The listing builds one solid part. Answer for the finished solid, in the listing's coordinates (mm). A direction names the side the tool comes from. Round coordinates to 2 decimals unless told otherwise and drop trailing zeros. Write each loop counter-clockwise with the first axis right and the second up, starting at its lowest first coordinate (ties: lowest second). Pieces come first, ordered by that corner, then holes.
(1) A cutting plane is placed at C-C, the plane y = 6. Give the vertices of the cut face in (x, z), and give its area (3 significant figures).
(2) For faces 4 (the face through (-2, 16.7, -3.5)), 5 (the face through (-3.4, 11.3, -5)), 6 (the face through (-8, 3.7, -4)), 7 (the face through (-7.5, 1.9, 6.5)), determine the directions among +Z, -Z, +X, -X, +Y, -Y from which every point of the face is accessible in a straight line to the end or side of a thin tool.
(3) A cutting plane is placed at D-D, the plane x = -1.75. Give the vertices of the cut face in (y, z), and give its area (3 significant figures).
(4) A cutting plane is placed at A-A, the plane z = 1.5. Give the vertices of the cut face in (x, y).
(5) Find the intervals of material crossed by probe 1 along X at (y, z) = (1.5, 1.25); probe 2 along X at (y, z) = (11.5, -4.25); probe 3 along X at (y, z) = (10, -5.5), in increasing order.
(6) Each of these flat-tipped pins is pushed along its axis until it touches: pin 1 Ø6.5 at (y, z) = (7.5, -5) entering from +X; pin 2 Ø3.5 at (x, y) = (-4.5, 12) entering from -Z; pin 3 Ø0.9 at (x, z) = (-7.5, -4) entering from -Y. Where does it stop, or does it pass through?
(7) A cutting plane is placed at B-B, the plane x = -7.5. Give the vertices of the cut face in (y, z).
(8) The mould has two halves that part along X. Classify faces 1 (the face through (6.55, 2, 0)), 2 (the face through (-4, 11, -2)), 3 (the face through (-10.5, 7, -3)): +X half, -X half, draft (parallel to the pull), parting line (faces both ways), or undercut.
from build123d import *

# Parameters (mm, degrees)
SKETCH1_W           = 10
SKETCH1_H           = 16
BOSS_EXTRUDE1_DEPTH = 3.7
SKETCH5_W           = 5.5
SKETCH5_H           = 16
BOSS_EXTRUDE2_DEPTH = 3.7
CUT_EXTRUDE4_DEPTH  = 4.7
BOSS_EXTRUDE3_START = -2
SKETCH7_W           = 17
SKETCH7_H           = 15
BOSS_EXTRUDE3_DEPTH = 3
SKETCH8_W           = 2.5
SKETCH8_H           = 15
BOSS_EXTRUDE5_DEPTH = 3


with BuildPart() as part:
    # Sketch1 → Boss-Extrude1 (new body)
    with BuildSketch(Plane(origin=(0, 0, 0), x_dir=(1, 0, 0), z_dir=(0, 1, 0))):
        Rectangle(SKETCH1_W, SKETCH1_H)
    extrude(amount=BOSS_EXTRUDE1_DEPTH)

    # Sketch5 → Boss-Extrude2 (add)
    with BuildSketch(Plane.XZ):
        with Locations((-7.75, 0)):
            Rectangle(SKETCH5_W, SKETCH5_H)
    boss_extrude2 = extrude(amount=-BOSS_EXTRUDE2_DEPTH)

    # Sketch6 → Cut-Extrude4 (cut, through all)
    with BuildSketch(Plane(origin=(0, 3.7, 0), x_dir=(1, 0, 0), z_dir=(0, 1, 0))):
        with BuildLine():
            Line((-6.55, 5.55), (-6.55, -5.55))
            ThreePointArc((-6.55, -5.55), (-7.5, -6.5), (-8.45, -5.55))
            Line((-8.45, -5.55), (-8.45, 5.55))
            ThreePointArc((-8.45, 5.55), (-7.5, 6.5), (-6.55, 5.55))
        make_face()
    cut_extrude4 = extrude(amount=-CUT_EXTRUDE4_DEPTH, mode=Mode.SUBTRACT)

    # Mirror1: Boss-Extrude2, Cut-Extrude4 across plane
    add(boss_extrude2.mirror(Plane(origin=(0, 0, 0), x_dir=(0, 0, 1), z_dir=(1, 0, 0))))
    add(cut_extrude4.mirror(Plane(origin=(0, 0, 0), x_dir=(0, 0, 1), z_dir=(1, 0, 0))), mode=Mode.SUBTRACT)



with BuildPart() as body_2:
    # Sketch7 → Boss-Extrude3 (new body)
    with BuildSketch(Plane.XY.offset(BOSS_EXTRUDE3_START)):
        with Locations((-2, 11.2)):
            Rectangle(SKETCH7_W, SKETCH7_H)
        with BuildLine():
            Line((-3, 15.7), (-3, 5.7))
            ThreePointArc((-3, 5.7), (-2, 4.7), (-1, 5.7))
            Line((-1, 5.7), (-1, 15.7))
            ThreePointArc((-1, 15.7), (-2, 16.7), (-3, 15.7))
        make_face(mode=Mode.SUBTRACT)
    extrude(amount=-BOSS_EXTRUDE3_DEPTH)


with BuildPart() as part_1:
    add(part.part)

    add(body_2.part)  # Boss-Extrude5 merges body 2
    # Sketch8 → Boss-Extrude5 (add)
    with BuildSketch(Plane(origin=(0, 0, -5), x_dir=(-1, 0, 0), z_dir=(0, 0, -1))):
        with Locations((-5.25, 11.2)):
            Rectangle(SKETCH8_W, SKETCH8_H)
        with Locations((9.25, 11.2)):
            Rectangle(SKETCH8_W, SKETCH8_H)
    extrude(amount=BOSS_EXTRUDE5_DEPTH)


solid = part_1.part
Solutions:
1. outline: (-10.5, -8) - (-8, -8) - (-8, -5) - (-3, -5) - (-3, -2) - (-10.5, -2) - close; (-1, -5) - (4, -5) - (4, -8) - (6.5, -8) - (6.5, -2) - (-1, -2) - close
1. area: 60.0 mm2
2. face 4: +Z, -Z
2. face 5: -Z, +Y
2. face 6: -Y
2. face 7: +Y, -Y
3. outline: (0, -8) - (3.7, -8) - (3.7, -5) - (4.73, -5) - (4.73, -2) - (3.7, -2) - (3.7, 8) - (0, 8) - close; (16.67, -5) - (18.7, -5) - (18.7, -2) - (16.67, -2) - close
3. area: 68.4 mm2
4. outline: (-10.5, 0) - (-8.45, 0) - (-8.45, 3.7) - (-10.5, 3.7) - close; (-6.55, 0) - (6.55, 0) - (6.55, 3.7) - (-6.55, 3.7) - close; (8.45, 0) - (10.5, 0) - (10.5, 3.7) - (8.45, 3.7) - close
5. probe 1: x = -10.5 to -8.45, -6.55 to 6.55, 8.45 to 10.5
5. probe 2: x = -10.5 to -3, -1 to 6.5
5. probe 3: x = -10.5 to -8, 4 to 6.5
6. pin 1: stops at x = 6.5
6. pin 2: stops at z = -5
6. pin 3: stops at y = 3.7
7. outline: (0, -8) - (3.7, -8) - (3.7, -6.5) - (0, -6.5) - close; (0, 6.5) - (3.7, 6.5) - (3.7, 8) - (0, 8) - close; (3.7, -5) - (18.7, -5) - (18.7, -2) - (3.7, -2) - close
8. face 1: undercut
8. face 2: draft
8. face 3: -X half
